```python
from build123d import *

# Parameters (mm, degrees)
SKETCH1_W           = 914.4
SKETCH1_H           = 812.8
SKETCH1_W_2         = 762
SKETCH1_H_2         = 660.4
BOSS_EXTRUDE1_DEPTH = 101.6
FILLET1_R           = 25.4
FILLET2_R           = 25.4
FILLET3_R           = 50.8


with BuildPart() as part:
    # Sketch1 → Boss-Extrude1 (new body)
    with BuildSketch(Plane(origin=(0, 0, 0), x_dir=(1, 0, 0), z_dir=(0, 1, 0))):
        with Locations((381, 330.2)):
            Rectangle(SKETCH1_W, SKETCH1_H)
        with Locations((381, 330.2)):
            Rectangle(SKETCH1_W_2, SKETCH1_H_2, mode=Mode.SUBTRACT)
    extrude(amount=BOSS_EXTRUDE1_DEPTH)

    # Fillet1
    fillet1_edges = [part.edges().sort_by_distance(p)[0] for p in [
        (381, 101.6, -736.6),
        (-76.2, 101.6, -330.2),
        (381, 101.6, 76.2),
        (838.2, 101.6, -330.2),
    ]]
    fillet(fillet1_edges, radius=FILLET1_R)

    # Fillet2
    fillet2_edges = [part.edges().sort_by_distance(p)[0] for p in [
        (-76.2, 0, -330.2),
        (381, 0, -736.6),
        (838.2, 0, -330.2),
        (381, 0, 76.2),
    ]]
    fillet(fillet2_edges, radius=FILLET2_R)

    # Fillet3
    # the kernel refuses this fillet: 50.8 mm, written as the material it takes off along each edge
    with BuildSketch(Plane(origin=(-25.4, 101.6, -685.8), x_dir=(0, 0, -1), z_dir=(1, 0, 0))) as fillet3_piece_1:
        with BuildLine():
            CenterArc((25.4, -25.4), 25.4, 0, 90)
            Line((50.8, -25.4), (50.8, 0))
            Line((50.8, 0), (25.4, 0))
        make_face()
    revolve(axis=Axis((-25.4, 101.6, -685.8), (0, 1, 0)), revolution_arc=90, mode=Mode.SUBTRACT)
    with BuildSketch(Plane(origin=(787.4, 101.6, -685.8), x_dir=(1, 0, 0), z_dir=(0, 0, 1))) as fillet3_piece_2:
        with BuildLine():
            CenterArc((25.4, -25.4), 25.4, 0, 90)
            Line((50.8, -25.4), (50.8, 0))
            Line((50.8, 0), (25.4, 0))
        make_face()
    revolve(axis=Axis((787.4, 101.6, -685.8), (0, 1, 0)), revolution_arc=90, mode=Mode.SUBTRACT)
    with BuildSketch(Plane(origin=(-25.4, 101.6, 25.4), x_dir=(-1, 0, 0), z_dir=(0, 0, -1))) as fillet3_piece_3:
        with BuildLine():
            CenterArc((25.4, -25.4), 25.4, 0, 90)
            Line((50.8, -25.4), (50.8, 0))
            Line((50.8, 0), (25.4, 0))
        make_face()
    revolve(axis=Axis((-25.4, 101.6, 25.4), (0, 1, 0)), revolution_arc=90, mode=Mode.SUBTRACT)
    with BuildSketch(Plane(origin=(787.4, 101.6, 25.4), x_dir=(0, 0, 1), z_dir=(-1, 0, 0))) as fillet3_piece_4:
        with BuildLine():
            CenterArc((25.4, -25.4), 25.4, 0, 90)
            Line((50.8, -25.4), (50.8, 0))
            Line((50.8, 0), (25.4, 0))
        make_face()
    revolve(axis=Axis((787.4, 101.6, 25.4), (0, 1, 0)), revolution_arc=90, mode=Mode.SUBTRACT)
    with BuildSketch(Plane(origin=(787.4, 0, 25.4), x_dir=(1, 0, 0), z_dir=(0, 0, -1))) as fillet3_piece_5:
        with BuildLine():
            CenterArc((25.4, -25.4), 25.4, 0, 90)
            Line((50.8, -25.4), (50.8, 0))
            Line((50.8, 0), (25.4, 0))
        make_face()
    revolve(axis=Axis((787.4, 0, 25.4), (0, -1, 0)), revolution_arc=90, mode=Mode.SUBTRACT)
    with BuildSketch(Plane(origin=(-25.4, 0, 25.4), x_dir=(0, 0, 1), z_dir=(1, 0, 0))) as fillet3_piece_6:
        with BuildLine():
            CenterArc((25.4, -25.4), 25.4, 0, 90)
            Line((50.8, -25.4), (50.8, 0))
            Line((50.8, 0), (25.4, 0))
        make_face()
    revolve(axis=Axis((-25.4, 0, 25.4), (0, -1, 0)), revolution_arc=90, mode=Mode.SUBTRACT)
    with BuildSketch(Plane(origin=(787.4, 0, -685.8), x_dir=(0, 0, -1), z_dir=(-1, 0, 0))) as fillet3_piece_7:
        with BuildLine():
            CenterArc((25.4, -25.4), 25.4, 0, 90)
            Line((50.8, -25.4), (50.8, 0))
            Line((50.8, 0), (25.4, 0))
        make_face()
    revolve(axis=Axis((787.4, 0, -685.8), (0, -1, 0)), revolution_arc=90, mode=Mode.SUBTRACT)
    with BuildSketch(Plane(origin=(-25.4, 0, -685.8), x_dir=(-1, 0, 0), z_dir=(0, 0, 1))) as fillet3_piece_8:
        with BuildLine():
            CenterArc((25.4, -25.4), 25.4, 0, 90)
            Line((50.8, -25.4), (50.8, 0))
            Line((50.8, 0), (25.4, 0))
        make_face()
    revolve(axis=Axis((-25.4, 0, -685.8), (0, -1, 0)), revolution_arc=90, mode=Mode.SUBTRACT)
    with BuildSketch(Plane(origin=(838.2, 0, 76.2), x_dir=(-1, 0, 0), z_dir=(0, 1, 0)), Plane(origin=(-76.2, 0, 76.2), x_dir=(0, 0, -1), z_dir=(0, 1, 0))) as fillet3_piece_9:
        with BuildLine():
            CenterArc((FILLET3_R, -FILLET3_R), FILLET3_R, 90, 90)
            Line((0, -FILLET3_R), (0, 0))
            Line((0, 0), (FILLET3_R, 0))
        make_face()
    extrude(amount=101.6, mode=Mode.SUBTRACT)
    with BuildSketch(Plane(origin=(838.2, 0, -736.6), x_dir=(-1, 0, 0), z_dir=(0, 1, 0)), Plane(origin=(-76.2, 0, -736.6), x_dir=(0, 0, 1), z_dir=(0, 1, 0))) as fillet3_piece_10:
        with BuildLine():
            CenterArc((FILLET3_R, FILLET3_R), FILLET3_R, 180, 90)
            Line((0, FILLET3_R), (0, 0))
            Line((0, 0), (FILLET3_R, 0))
        make_face()
    extrude(amount=101.6, mode=Mode.SUBTRACT)


solid = part.part
```
Geometry: final body of the model. Coordinates: model frame, mm. A direction names the side the tool comes from. Round coordinates to 2 decimals unless told otherwise and drop trailing zeros. Write each loop counter-clockwise with the first axis right and the second up, starting at its lowest first coordinate (ties: lowest second). Pieces come first, ordered by that corner, then holes. Notation, with made-up numbers: M 88,49 L 109,49 A12 ccw 109,61 Z; hole C 20.25,26.5 d3. An arc over 180 degrees is marked long. Answer in a Markdown table with one row per item. Add a question column.
(1) Cut plane A-A, the plane z = -113. Return the cut outline in (x, y).
(2) Draft query along X for faces 3 (the face through (375, 50, 76.2)), 4 (the face through (830.96, 93.96, -335.18)), 5 (the face through (-68.96, 7.64, -335.18)), 6 (the face through (376, 50, 0)). Return one class per face: pulls with the +X half, pulls with the -X half, needs draft (parallel to the pull), parting line crosses it, or undercut.
(3) Ray query, L1, parallel to Z at x = 376, y = 36; L2, parallel to X at y = 51.5, z = -623.5; L3, parallel to X at y = 78, z = -323. Return the intervals inside material, ascending.
(4) Cut plane B-B, the plane x = 273.5. Return the cut outline in (y, z).
(5) Reachability of faces 1 (the face through (386.69, 93.96, -729.36)), 2 (the face through (762, 50, -326)) from +Z, -Z, +X, -X, +Y, -Y: full face, straight path, thin tool, end or side. Return the list, or none.
(6) Contact query for flat-ended pins moving along their axis: pin 1 (4 mm diameter, centred on y = 89, z = -157.5, fed in from -X); pin 2 (8 mm diameter, centred on y = 86.5, z = -77.5, fed in from -X); pin 3 (12 mm diameter, centred on y = 15.5, z = -375, fed in from -X). Output: stop coordinate, or through.
Established:
| question | item | result |
|---|---|---|
| 1 | outline | M -76.2,25.4 A25.4 ccw -50.8,0 L 0,0 L 0,101.6 L -50.8,101.6 A25.4 ccw -76.2,76.2 Z; M 762,0 L 812.8,0 A25.4 ccw 838.2,25.4 L 838.2,76.2 A25.4 ccw 812.8,101.6 L 762,101.6 Z |
| 2 | face 3 | needs draft |
| 2 | face 4 | pulls with the +X half |
| 2 | face 5 | pulls with the -X half |
| 2 | face 6 | undercut |
| 3 | L1 | -736.6 to -660.4, 0 to 76.2 |
| 3 | L2 | -76.2 to 0, 762 to 838.2 |
| 3 | L3 | -76.14 to 0, 762 to 838.14 |
| 4 | outline | M 0,-711.2 A25.4 ccw 25.4,-736.6 L 76.2,-736.6 A25.4 ccw 101.6,-711.2 L 101.6,-660.4 L 0,-660.4 Z; M 0,0 L 101.6,0 L 101.6,50.8 A25.4 ccw 76.2,76.2 L 25.4,76.2 A25.4 ccw 0,50.8 Z |
| 5 | face 1 | -Z, +X, -X, +Y |
| 5 | face 2 | +Y, -Y |
| 6 | pin 1 | x = -73.79 |
| 6 | pin 2 | x = -75.41 |
| 6 | pin 3 | x = -75.9 |
